Design review of the part built by this model. Coordinates are the model's own, in mm. A direction names the side the tool comes from. Coordinates: 2 decimals unless noted, no trailing zeros. Write each loop counter-clockwise with the first axis right and the second up, starting at its lowest first coordinate (ties: lowest second). Pieces come first, ordered by that corner, then holes. Notation, with made-up numbers: (28, -33) -> (72, -33) arc R21 cw to (72, -7) -> close; hole circle Ø3 at (71.5, 49). An arc over 180 degrees is marked (long way). Answer in a Markdown table with one row per item. Add a question column.
Item 1: For faces 1 (the face through (52.683, 25.829, 1.479)), 2 (the face through (1.134, 5.786, 1.479)), 3 (the face through (2, -1, 6)), 4 (the face through (30.017, 13.571, 1.479)), 5 (the face through (-0.867, -3.905, 4.479)), list the 3-axis set-ups (+Z, -Z, +X, -X, +Y, -Y) from which the entire face can be reached by the end or side of a thin tool; tool diameter is ignored.
Item 2: Take a section at C-C, the plane x = 10. Write out the cut boundary in (y, z), and give its area (3 significant figures).
Item 3: To check wall thickness, follow line 1 (Y direction, x = 0, z = 3.1); line 2 (Z direction, x = 37, y = 17.5); line 3 (Y direction, x = 25, z = 0.75). State the ranges of each line that lie inside material, in increasing order.
Item 4: Draft analysis for pull direction X (two halves, no side actions). For faces 6 (the face through (39.385, 39.749, 1.479)), 7 (the face through (-4.168, 3.109, 1.479)), 8 (the face through (29, 10, 0)), 9 (the face through (29.624, 36.621, 1.479)), state which applies: released by +X, released by -X, zero draft, split by the parting line, or undercut.
Item 5: Take a section at A-A, the plane z = 4.75. Write out the cut boundary in (x, y), and give its area (3 significant figures).
Item 6: Take a section at B-B, the plane y = 20. Write out the cut boundary in (x, z).
Item 7: Clearance check with flat-ended pins moving along their axes: P1, Ø1, axis at x = 35.5, y = 1.5, coming from the +Z side; P2, Ø12, axis at x = 21.5, y = 22, coming from the +Z side; P3, Ø1.5, axis at y = 44, z = 1.5, coming from the +X side; P4, Ø1.5, axis at y = 29.5, z = 2.5, coming from the -X side. State where each tip first meets the part, or that it passes through.
from build123d import *

# Parameters (mm, degrees)
PAD_DEPTH                                 = 3
EXTRUDE_DEPTH                             = 3
EXTRUDE_ONTO_INVOLUTEGEAR_PLACEMENT_ANGLE = -15
EXTRUDE_PLACEMENT_ANGLE                   = 29.533929
SKETCH001_R                               = 4
PAD001_DEPTH                              = 3
SKETCH002_R                               = 1.75
POCKET001_DEPTH                           = 6.001


with BuildPart() as claw_body:
    # Sketch → Pad (new body)
    with BuildSketch(Plane.XY):
        with BuildLine():
            ThreePointArc((2.197615, -4.7128), (3.983431, 3.342496), (-4.259591, 2.982597))
            Line((-5.488319, 3.842962), (-4.259591, 2.982597))
            Line((-5.488319, 3.842962), (-21.76598, 2.989886))
            ThreePointArc((-22.627333, 3.40073), (-22.248827, 3.08593), (-21.76598, 2.989886))
            Line((-22.627333, 3.40073), (-37.615857, 24.030664))
            ThreePointArc((-37.625992, 25.192025), (-37.806802, 24.609722), (-37.615857, 24.030664))
            Line((-37.625992, 25.192025), (-21.393779, 48.374028))
            ThreePointArc((-21.393779, 48.374028), (-21.125112, 49.710122), (-21.924071, 50.814201))
            ThreePointArc((-21.924071, 50.814201), (-25.071791, 51.496726), (-28.008332, 50.173585))
            Line((-28.008332, 50.173585), (-51.085112, 29.027611))
            ThreePointArc((-51.085112, 29.027611), (-52.688135, 25.777003), (-51.673928, 22.297417))
            Line((-51.673928, 22.297417), (-26.288576, -10.785417))
            ThreePointArc((-26.288576, -10.785417), (-24.440562, -12.203448), (-22.131119, -12.507492))
            Line((-22.131119, -12.507492), (-0.517621, -9.662021))
            ThreePointArc((-0.517621, -9.662021), (2.094081, -7.875425), (2.197615, -4.7128))
        make_face()
    extrude(amount=PAD_DEPTH)


with BuildPart() as part_mirroring:
    # Part__Mirroring: instance of claw-body
    add(claw_body.part.mirror(Plane(origin=(0, 0, 0), x_dir=(0, -1, 0), z_dir=(1, 0, 0))))


with BuildPart() as drill:
    # InvoluteGear as drawn → Extrude (new)
    with BuildSketch(Plane.XY):
        with BuildLine():
            Line((4.810602, -1.107072), (6.405135, -1.472675))
            add(Edge.make_bspline(
                [(6.405135, -1.472675), (6.508382, -1.483345), (6.922829, -1.512197), (7.670072, -1.341281), (8.519169, -0.723794)],
                knots=[0, 0, 0, 0, 0, 1, 1, 1, 1, 1], degree=4))
            ThreePointArc((8.519169, -0.723794), (8.54986, 0), (8.519169, 0.723794))
            add(Edge.make_bspline(
                [(8.519169, 0.723794), (7.670072, 1.341281), (6.922829, 1.512197), (6.508382, 1.483345), (6.405135, 1.472675)],
                knots=[0, 0, 0, 0, 0, 1, 1, 1, 1, 1], degree=4))
            Line((6.405135, 1.472675), (4.810602, 1.107072))
            ThreePointArc((4.810602, 1.107072), (4.31977, 1.170473), (3.988644, 1.538293))
            ThreePointArc((3.988644, 1.538293), (3.851642, 1.854853), (3.689565, 2.159338))
            ThreePointArc((3.689565, 2.159338), (3.608445, 2.647554), (3.864905, 3.070832))
            Line((3.864905, 3.070832), (5.14492, 4.089539))
            add(Edge.make_bspline(
                [(5.14492, 4.089539), (5.217636, 4.163608), (5.498597, 4.469646), (5.830867, 5.160429), (5.8775, 6.209276)],
                knots=[0, 0, 0, 0, 0, 1, 1, 1, 1, 1], degree=4))
            ThreePointArc((5.8775, 6.209276), (5.330751, 6.68455), (4.74573, 7.111832))
            add(Edge.make_bspline(
                [(4.74573, 7.111832), (3.733556, 6.832978), (3.13403, 6.355326), (2.898184, 6.013309), (2.842153, 5.925934)],
                knots=[0, 0, 0, 0, 0, 1, 1, 1, 1, 1], degree=4))
            Line((2.842153, 5.925934), (2.133817, 4.451328))
            ThreePointArc((2.133817, 4.451328), (1.77822, 4.10711), (1.284193, 4.077557))
            ThreePointArc((1.284193, 4.077557), (0.951277, 4.167817), (0.612168, 4.230943))
            ThreePointArc((0.612168, 4.230943), (0.179887, 4.471919), (0.008856, 4.936337))
            Line((0.008856, 4.936337), (0.010475, 6.572246))
            add(Edge.make_bspline(
                [(0.010475, 6.572246), (-0.002097, 6.675279), (-0.066191, 7.085755), (-0.3991, 7.77623), (-1.190047, 8.466635)],
                knots=[0, 0, 0, 0, 0, 1, 1, 1, 1, 1], degree=4))
            ThreePointArc((-1.190047, 8.466635), (-1.902523, 8.335497), (-2.60134, 8.144516))
            add(Edge.make_bspline(
                [(-2.60134, 8.144516), (-3.014403, 7.179304), (-3.014758, 6.412764), (-2.894406, 6.015128), (-2.861029, 5.916844)],
                knots=[0, 0, 0, 0, 0, 1, 1, 1, 1, 1], degree=4))
            Line((-2.861029, 5.916844), (-2.149775, 4.443643))
            ThreePointArc((-2.149775, 4.443643), (-2.102366, 3.951009), (-2.387281, 3.546338))
            ThreePointArc((-2.387281, 3.546338), (-2.665419, 3.34233), (-2.926204, 3.116562))
            ThreePointArc((-2.926204, 3.116562), (-3.384129, 2.928837), (-3.853862, 3.08468))
            Line((-3.853862, 3.08468), (-5.131858, 4.105918))
            add(Edge.make_bspline(
                [(-5.131858, 4.105918), (-5.220251, 4.160329), (-5.581136, 4.366146), (-6.328536, 4.536371), (-7.361464, 4.348444)],
                knots=[0, 0, 0, 0, 0, 1, 1, 1, 1, 1], degree=4))
            ThreePointArc((-7.361464, 4.348444), (-7.703158, 3.709645), (-7.989548, 3.044213))
            add(Edge.make_bspline(
                [(-7.989548, 3.044213), (-7.492456, 2.119467), (-6.893372, 1.64126), (-6.507449, 1.487434), (-6.409797, 1.45225)],
                knots=[0, 0, 0, 0, 0, 1, 1, 1, 1, 1], degree=4))
            Line((-6.409797, 1.45225), (-4.814543, 1.089804))
            ThreePointArc((-4.814543, 1.089804), (-4.399827, 0.819718), (-4.261084, 0.344654))
            ThreePointArc((-4.261084, 0.344654), (-4.275, 0), (-4.261084, -0.344654))
            ThreePointArc((-4.261084, -0.344654), (-4.399827, -0.819718), (-4.814543, -1.089804))
            Line((-4.814543, -1.089804), (-6.409797, -1.45225))
            add(Edge.make_bspline(
                [(-6.409797, -1.45225), (-6.507449, -1.487434), (-6.893372, -1.64126), (-7.492456, -2.119467), (-7.989548, -3.044213)],
                knots=[0, 0, 0, 0, 0, 1, 1, 1, 1, 1], degree=4))
            ThreePointArc((-7.989548, -3.044213), (-7.703158, -3.709645), (-7.361464, -4.348444))
            add(Edge.make_bspline(
                [(-7.361464, -4.348444), (-6.328536, -4.536371), (-5.581136, -4.366146), (-5.220251, -4.160329), (-5.131858, -4.105918)],
                knots=[0, 0, 0, 0, 0, 1, 1, 1, 1, 1], degree=4))
            Line((-5.131858, -4.105918), (-3.853862, -3.08468))
            ThreePointArc((-3.853862, -3.08468), (-3.384129, -2.928837), (-2.926204, -3.116562))
            ThreePointArc((-2.926204, -3.116562), (-2.665419, -3.34233), (-2.387281, -3.546338))
            ThreePointArc((-2.387281, -3.546338), (-2.102366, -3.951009), (-2.149775, -4.443643))
            Line((-2.149775, -4.443643), (-2.861029, -5.916844))
            add(Edge.make_bspline(
                [(-2.861029, -5.916844), (-2.894406, -6.015128), (-3.014758, -6.412764), (-3.014403, -7.179304), (-2.60134, -8.144516)],
                knots=[0, 0, 0, 0, 0, 1, 1, 1, 1, 1], degree=4))
            ThreePointArc((-2.60134, -8.144516), (-1.902523, -8.335497), (-1.190047, -8.466635))
            add(Edge.make_bspline(
                [(-1.190047, -8.466635), (-0.3991, -7.77623), (-0.066191, -7.085755), (-0.002097, -6.675279), (0.010475, -6.572246)],
                knots=[0, 0, 0, 0, 0, 1, 1, 1, 1, 1], degree=4))
            Line((0.010475, -6.572246), (0.008856, -4.936337))
            ThreePointArc((0.008856, -4.936337), (0.179887, -4.471919), (0.612168, -4.230943))
            ThreePointArc((0.612168, -4.230943), (0.951277, -4.167817), (1.284193, -4.077557))
            ThreePointArc((1.284193, -4.077557), (1.77822, -4.10711), (2.133817, -4.451328))
            Line((2.133817, -4.451328), (2.842153, -5.925934))
            add(Edge.make_bspline(
                [(2.842153, -5.925934), (2.898184, -6.013309), (3.13403, -6.355326), (3.733556, -6.832978), (4.74573, -7.111832)],
                knots=[0, 0, 0, 0, 0, 1, 1, 1, 1, 1], degree=4))
            ThreePointArc((4.74573, -7.111832), (5.330751, -6.68455), (5.8775, -6.209276))
            add(Edge.make_bspline(
                [(5.8775, -6.209276), (5.830867, -5.160429), (5.498597, -4.469646), (5.217636, -4.163608), (5.14492, -4.089539)],
                knots=[0, 0, 0, 0, 0, 1, 1, 1, 1, 1], degree=4))
            Line((5.14492, -4.089539), (3.864905, -3.070832))
            ThreePointArc((3.864905, -3.070832), (3.608445, -2.647554), (3.689565, -2.159338))
            ThreePointArc((3.689565, -2.159338), (3.851642, -1.854853), (3.988644, -1.538293))
            ThreePointArc((3.988644, -1.538293), (4.31977, -1.170473), (4.810602, -1.107072))
        make_face()
    extrude(amount=EXTRUDE_DEPTH)


with BuildPart() as drill_1:
    # Extrude onto InvoluteGear placement: moved
    add(drill.part.rotate(Axis((0, 0, 0), (0, 0, 1)), EXTRUDE_ONTO_INVOLUTEGEAR_PLACEMENT_ANGLE))


with BuildPart() as drill_2:
    # Extrude placement: moved
    add(drill_1.part.rotate(Axis((0, 0, 0), (0, 0, 1)), EXTRUDE_PLACEMENT_ANGLE))

    # Fusion001: union Part__Mirroring
    add(part_mirroring.part)

    # Sketch001 → Pad001 (new body)
    with BuildSketch(Plane.XY.offset(3)):
        Circle(SKETCH001_R)
    extrude(amount=PAD001_DEPTH)

    # Sketch002 → Pocket001 (cut, through all)
    with BuildSketch(Plane.XY.offset(6)):
        Circle(SKETCH002_R)
    extrude(amount=-POCKET001_DEPTH, mode=Mode.SUBTRACT)


solid = drill_2.part
Answers:
| question | item | result |
|---|---|---|
| 1 | face 1 | +Z, -Z, +X |
| 1 | face 2 | +Z, -Z, +Y |
| 1 | face 3 | +Z, +X, -X, +Y, -Y |
| 1 | face 4 | +Z, -Z |
| 1 | face 5 | +Z |
| 2 | outline | (-10.91, 0) -> (3.61, 0) -> (3.61, 3) -> (-10.91, 3) -> close |
| 2 | area | 43.6 mm^2 |
| 3 | line 1 | y = -4 to -1.75, 1.75 to 4 |
| 3 | line 2 | z = 0 to 3 |
| 3 | line 3 | y = -11.92 to 6.67, 43.22 to 51.5 |
| 4 | face 6 | released by +X |
| 4 | face 7 | undercut |
| 4 | face 8 | zero draft |
| 4 | face 9 | released by -X |
| 5 | outline | circle Ø8 at (0, 0); hole circle Ø3.5 at (0, 0) |
| 5 | area | 40.6 mm^2 |
| 6 | outline | (34.69, 0) -> (49.91, 0) -> (49.91, 3) -> (34.69, 3) -> close |
| 7 | P1 | stops at z = 3 |
| 7 | P2 | passes through |
| 7 | P3 | stops at x = 35.56 |
| 7 | P4 | stops at x = 34.08 |
